```python
from build123d import *

# Parameters (mm, degrees)
F0_W     = 378.7394
F0_H     = 751.84
F0_H_2   = 10.16
F1_DEPTH = 2.54
F2_W     = 327.9394
F2_H     = 152.4
F2_H_2   = 558.8
F2_R     = 3.175
F3_DEPTH = 2.541


# Not quite as in the source:
# - a length typed as a fraction of an inch, garbled in the dataset ("3 / 203.2 mm" for 3/8 in), is restored


with BuildPart() as f1:
    # F0 (on Front) → F1 (new body)
    with BuildSketch(Plane.XZ):
        with Locations((0, -5.08)):
            Rectangle(F0_W, F0_H)
        with Locations((0, 375.92)):
            Rectangle(F0_W, F0_H_2)
    extrude(amount=F1_DEPTH)

    # F2 (on face) → F3 (cut, through all)
    with BuildSketch(Plane.XZ.offset(2.54)):
        with Locations((0, -304.8)):
            Rectangle(F2_W, F2_H)
        with Locations((0, 76.2)):
            Rectangle(F2_W, F2_H_2)
        with BuildLine():
            ThreePointArc((178.1250186398, 307.6218208052), (173.9584953156, 303.1477306033), (179.8447, 304.8))
            ThreePointArc((179.8447, 304.8), (179.3809046844, 306.4522693967), (178.1250186398, 307.6218208052))
        make_face()
        with BuildLine():
            ThreePointArc((176.6697, -149.225), (174.4246359697, -154.6450640303), (179.8447, -152.4))
            ThreePointArc((179.8447, -152.4), (178.9147640303, -150.1549359697), (176.6697, -149.225))
        make_face()
        with BuildLine():
            ThreePointArc((-176.6697, -149.225), (-178.9147640303, -154.6450640303), (-173.4947, -152.4))
            ThreePointArc((-173.4947, -152.4), (-174.4246359697, -150.1549359697), (-176.6697, -149.225))
        make_face()
        with Locations((-176.6697, 304.8)):
            Circle(F2_R)
    extrude(amount=-F3_DEPTH, mode=Mode.SUBTRACT)


solid = f1.part
```
Work out the finished part from the listing and answer in its coordinate system (mm). Give positions to 0.01 mm unless a question says otherwise; leave off trailing zeros. Write each loop counter-clockwise with the first axis right and the second up, starting at its lowest first coordinate (ties: lowest second). Pieces come first, ordered by that corner, then holes.
(1) The part is cut by section C-C on y = -0.65. Write down the section's boundary in (x, z) (3 decimals).
Final values:
outline: (-189.37, -381) - (-163.97, -381) - (-163.97, -228.6) - (163.97, -228.6) - (163.97, -381) - (189.37, -381) - (189.37, 381) - (-189.37, 381) - close; hole circle Ø6.35 at (-176.67, -152.4); hole circle Ø6.35 at (-176.67, 304.8); hole (-163.97, -203.2) - (163.97, -203.2) - (163.97, 355.6) - (-163.97, 355.6) - close; hole circle Ø6.35 at (176.67, -152.4); hole circle Ø6.35 at (176.67, 304.8)
(2) Straight lines are drawn through the part: line 1 (X direction, y = -1.3, z = -152.4); line 2 (X direction, y = -1.55, z = 112); line 3 (Z direction, x = -147.5, y = -0.9). For each, find the intervals that lie inside material, in ascending order.
Final values:
line 1: x = -189.37 to -179.84, -173.49 to -163.97, 163.97 to 173.49, 179.84 to 189.37
line 2: x = -189.37 to -163.97, 163.97 to 189.37
line 3: z = -228.6 to -203.2, 355.6 to 381
(3) The part is cut by section B-B on x = -119.5. Write down the section's boundary in (y, z), plus the area to 3 significant figures.
Final values:
outline: (-2.54, -228.6) - (0, -228.6) - (0, -203.2) - (-2.54, -203.2) - close; (-2.54, 355.6) - (0, 355.6) - (0, 381) - (-2.54, 381) - close
area: 129 mm2
(4) A flat-ended cylindrical pin translates along its axis: pin 1 Ø1.3 at (x, y) = (-35.5, -2) entering from -Z. Find the tip coordinate at first contact, or state that the pin passes through.
Final values:
pin 1: stops at z = -228.6
(5) The part is cut by section A-A on z = -102. Write down the section's boundary in (x, y).
Final values:
outline: (-189.37, -2.54) - (-163.97, -2.54) - (-163.97, 0) - (-189.37, 0) - close; (163.97, -2.54) - (189.37, -2.54) - (189.37, 0) - (163.97, 0) - close
